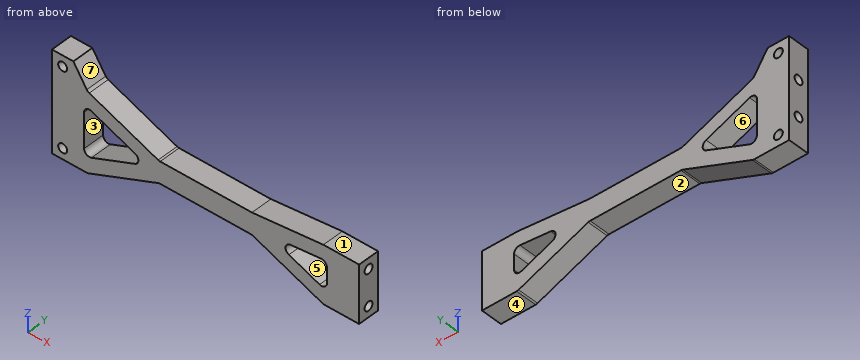
```python
from build123d import *

# Parameters (mm, degrees)
BOSS_EXTRUDE1_DEPTH         = 6
TAP_DRILL_FOR_M3_TAP3_D     = 2.5
TAP_DRILL_FOR_M3_TAP3_DEPTH = 10
TAP_DRILL_FOR_M3_TAP3_TIP   = 0.751075774
TAP_DRILL_FOR_M3_TAP2_D     = 2.5
TAP_DRILL_FOR_M3_TAP2_DEPTH = 8
TAP_DRILL_FOR_M3_TAP2_TIP   = 0.751075774
TAP_DRILL_FOR_M3_TAP1_D     = 2.5
TAP_DRILL_FOR_M3_TAP1_DEPTH = 8
TAP_DRILL_FOR_M3_TAP1_TIP   = 0.751075774
FILLET1_R                   = 1.5


with BuildPart() as part:
    # Sketch2 → Boss-Extrude1 (new body)
    with BuildSketch(Plane(origin=(0, 0, 0), x_dir=(1, 0, 0), z_dir=(0, 1, 0))):
        Polygon((56, -8), (76, 0), (86, 0), (86, -16), (76, -16), (56, -14), (30, -14), (10, -22), (6, -28), (0, -28), (0, 0), (10, 0), (30, -8), align=None)
        Polygon((9, -3.908131846), (26.729670386, -11), (9, -18.091868154), align=None, mode=Mode.SUBTRACT)
        Polygon((60.656164188, -10.44566617), (77, -12.080049752), (77, -3.908131846), align=None, mode=Mode.SUBTRACT)
    extrude(amount=BOSS_EXTRUDE1_DEPTH)

    # Tap Drill for M3 Tap3
    with Locations(Plane(origin=(0, 6, 0), x_dir=(1, 0, 0), z_dir=(0, 1, 0))):
        with Locations((3, -3), (3, -25)):
            Hole(TAP_DRILL_FOR_M3_TAP3_D / 2, depth=TAP_DRILL_FOR_M3_TAP3_DEPTH)
            with Locations((0, 0, -(TAP_DRILL_FOR_M3_TAP3_DEPTH + TAP_DRILL_FOR_M3_TAP3_TIP / 2))):  # 118° drill point
                Cone(0, TAP_DRILL_FOR_M3_TAP3_D / 2, TAP_DRILL_FOR_M3_TAP3_TIP, mode=Mode.SUBTRACT)

    # Tap Drill for M3 Tap2
    with Locations(Plane(origin=(86, 0.779165189, 7.640466368), x_dir=(0, 0, -1), z_dir=(1, 0, 0))):
        with Locations((-5.359533632, 2.220834811), (4.640466368, 2.220834811)):
            Hole(TAP_DRILL_FOR_M3_TAP2_D / 2, depth=TAP_DRILL_FOR_M3_TAP2_DEPTH)
            with Locations((0, 0, -(TAP_DRILL_FOR_M3_TAP2_DEPTH + TAP_DRILL_FOR_M3_TAP2_TIP / 2))):  # 118° drill point
                Cone(0, TAP_DRILL_FOR_M3_TAP2_D / 2, TAP_DRILL_FOR_M3_TAP2_TIP, mode=Mode.SUBTRACT)

    # Tap Drill for M3 Tap1
    with Locations(Plane.ZY):
        with Locations((8, 3), (18, 3)):
            Hole(TAP_DRILL_FOR_M3_TAP1_D / 2, depth=TAP_DRILL_FOR_M3_TAP1_DEPTH)
            with Locations((0, 0, -(TAP_DRILL_FOR_M3_TAP1_DEPTH + TAP_DRILL_FOR_M3_TAP1_TIP / 2))):  # 118° drill point
                Cone(0, TAP_DRILL_FOR_M3_TAP1_D / 2, TAP_DRILL_FOR_M3_TAP1_TIP, mode=Mode.SUBTRACT)

    # Fillet1
    fillet1_edges = [part.edges().sort_by_distance(p)[0] for p in [
        (10, 3, 0),
        (30, 3, 8),
        (56, 3, 8),
        (76, 3, 0),
        (30, 3, 14),
        (10, 3, 22),
        (9, 3, 18.091868154),
        (26.729670386, 3, 11),
        (9, 3, 3.908131846),
        (77, 3, 3.908131846),
        (60.656164188, 3, 10.44566617),
        (77, 3, 12.080049752),
    ]]
    fillet(fillet1_edges, radius=FILLET1_R)


solid = part.part
```
Read the model definition and answer for the solid it produces. Units are mm, in the model's axes. Face numbers are marked on the shaded views. A direction names the side the tool comes from. Round coordinates to 2 decimals unless told otherwise and drop trailing zeros. Write each loop counter-clockwise with the first axis right and the second up, starting at its lowest first coordinate (ties: lowest second). Pieces come first, ordered by that corner, then holes. Notation, with made-up numbers: (-10.75, 36.5) - (35.25, 36.5) arc R15 cw to (35.25, 57.5) - close; hole circle Ø1 at (4, -24). An arc over 180 degrees is marked (long way). One line per item, written item: value.
Q1. Find section A-A (x = 3). Determine the outline of the cut face in (y, z).
The answers:
outline: (0, 0) - (6, 0) - (6, 1.75) - (0, 1.75) - close; (0, 4.25) - (6, 4.25) - (6, 23.75) - (0, 23.75) - close; (0, 26.25) - (6, 26.25) - (6, 28) - (0, 28) - close; hole circle Ø2.5 at (3, 8); hole circle Ø2.5 at (3, 18)
Q2. For a pull along Z with two mould halves and no side action, classify the marked faces 4, 5, 6 and 7 as pulls with the +Z half, pulls with the -Z half, needs draft (parallel to the pull), parting line crosses it, or undercut.
The answers:
face 4: pulls with the -Z half
face 5: undercut
face 6: undercut
face 7: pulls with the +Z half
Q3. Straight lines are drawn through the part: line 1 (Z direction, x = 3, y = 4.5); line 2 (Z direction, x = 80.5, y = 3); line 3 (Y direction, x = 81.5, z = 3). For each, find the intervals that lie inside material, in ascending order. Write a range as from..to.
The answers:
line 1: z = 0..1.75, 4.25..23.75, 26.25..28
line 2: z = 0..1.75, 4.25..11.75, 14.25..16
line 3: y = 0..1.75, 4.25..6
Q4. Find section B-B (z = 25). Determine the outline of the cut face in (x, y).
The answers:
outline: (0, 0) - (1.75, 0) - (1.75, 6) - (0, 6) - close; (4.25, 0) - (8, 0) - (8, 6) - (4.25, 6) - close
Q5. Find section C-C (x = 80.5). Determine the outline of the cut face in (y, z).
The answers:
outline: (0, 0) - (6, 0) - (6, 16) - (0, 16) - close; hole circle Ø2.5 at (3, 3); hole circle Ø2.5 at (3, 13)
Q6. Which of the six approach directions +Z, -Z, +X, -X, +Y, -Y give full straight-line access (tool end or side, diameter ignored) to the marked faces 1, 2 and 3?
The answers:
face 1: +Z, +X, +Y, -Y
face 2: -Z, +Y, -Y
face 3: +Y, -Y
Q7. Each of these flat-tipped pins is pushed along its axis until it touches: P1, Ø3, axis at x = 3, z = 25, coming from the -Y side; P2, Ø5, axis at x = 59.5, z = 3, coming from the +Y side; P3, Ø1.8, axis at x = 47, y = 1.5, coming from the -Z side; P4, Ø1.5, axis at x = 10.5, y = 4.5, coming from the +Z side. Where does it stop, or does it pass through?
The answers:
P1: stops at y = 0
P2: passes through
P3: stops at z = 8
P4: stops at z = 22.38
Q8. Find section D-D (x = 17). Determine the outline of the cut face in (y, z), and give its area (3 significant figures).
The answers:
outline: (0, 2.8) - (6, 2.8) - (6, 7.11) - (0, 7.11) - close; (0, 14.89) - (6, 14.89) - (6, 19.2) - (0, 19.2) - close
area: 51.7 mm2
